Build history of the part. All positions in model axes, mm. A direction names the side the tool comes from. Give positions to 0.01 mm unless a question says otherwise; leave off trailing zeros. Write each loop counter-clockwise with the first axis right and the second up, starting at its lowest first coordinate (ties: lowest second). Pieces come first, ordered by that corner, then holes.
from build123d import *

# Parameters (mm, degrees)
SKETCH1_R           = 14.605
BOSS_EXTRUDE1_DEPTH = 1.524
CUT_EXTRUDE1_DEPTH  = 0.8128
SKETCH4_R           = 0.4445
BOSS_EXTRUDE2_DEPTH = 0.8128
CUT_EXTRUDE2_DEPTH  = 21.670575557
FILLET1_R           = 0.254
FILLET3_R           = 0.254
SNAP_START          = 13.7414
SNAP_HOOK1_DEPTH    = 0.6096
SNAP_START_2        = -0.714869456
SNAP_HOOK1_2_DEPTH  = 1.429738912
SNAP_START_3        = -0.847985215
SNAP_HOOK1_3_DEPTH  = 1.69597043
SNAP_START_4        = 12
SNAP_HOOK1_4_DEPTH  = 4
CIRPATTERN1_COUNT   = 4
SKETCH6_W           = 14.224
SKETCH6_H           = 9.208016637
CUT_EXTRUDE3_DEPTH  = 2.54


with BuildPart() as part:
    # Sketch1 → Boss-Extrude1 (new body)
    with BuildSketch(Plane(origin=(0, 0, 0), x_dir=(1, 0, 0), z_dir=(0, 1, 0))):
        with Locations(Location((0, 0, 0), (0, 0, 270))):
            Circle(SKETCH1_R)
    extrude(amount=BOSS_EXTRUDE1_DEPTH)

    # Sketch3 → Cut-Extrude1 (cut)
    with BuildSketch(Plane(origin=(0, 1.524, 0), x_dir=(1, 0, 0), z_dir=(0, 1, 0))):
        with BuildLine():
            Line((-5.588, -11.967686493), (5.588, -11.967686493))
            ThreePointArc((5.588, -11.967686493), (0, 13.208), (-5.588, -11.967686493))
        make_face()
    extrude(amount=-CUT_EXTRUDE1_DEPTH, mode=Mode.SUBTRACT)

    # Sketch4 → Boss-Extrude2 (add)
    with BuildSketch(Plane(origin=(0, 0.7112, 0), x_dir=(1, 0, 0), z_dir=(0, 1, 0))):
        with Locations(Location((-3.7592, -8.6233, 0), (0, 0, 90))):
            Circle(SKETCH4_R)
        with Locations(Location((3.7592, -8.6233, 0), (0, 0, 90))):
            Circle(SKETCH4_R)
    extrude(amount=BOSS_EXTRUDE2_DEPTH)

    # Sketch5 → Cut-Extrude2 (cut, through all)
    with BuildSketch(Plane(origin=(0, 0.7112, 0), x_dir=(1, 0, 0), z_dir=(0, 1, 0))):
        with BuildLine():
            Line((-9.940854815, -6.887686493), (9.870656967, -6.887686493))
            ThreePointArc((9.870656967, -6.887686493), (-0.035098924, 12.065), (-9.940854815, -6.887686493))
        make_face()
    extrude(amount=-CUT_EXTRUDE2_DEPTH, mode=Mode.SUBTRACT)

    # Fillet1
    fillet1_edges = [part.edges().sort_by_distance(p)[0] for p in [
        (-0.035098924, 0, -12.065),
        (-0.035098924, 0, 6.887686493),
    ]]
    fillet(fillet1_edges, radius=FILLET1_R)

    # Fillet3
    fillet3_edges = [part.edges().sort_by_distance(p)[0] for p in [
        (-3.7592, 1.524, 9.0678),
        (3.7592, 1.524, 9.0678),
    ]]
    fillet(fillet3_edges, radius=FILLET3_R)

    # Snap Hook1: read off the stored shape, not the designer's step
    # Snap Hook1 outline → Snap Hook1 (add)
    with BuildSketch(Plane.XY.offset(SNAP_START)):
        Polygon((-0.847985215, 1.524), (0.847985215, 1.524), (0.635, 5.588), (-0.635, 5.588), align=None)
    snap_hook1 = extrude(amount=SNAP_HOOK1_DEPTH)

    # Snap Hook1 2 outline → Snap Hook1 2 (add)
    with BuildSketch(Plane.YZ.offset(SNAP_START_2)):
        Polygon((1.524, 13.7414), (1.524, 13.335), (5.588, 13.7414), align=None)
        Polygon((4.064, 15.113), (4.064, 14.351), (5.588, 14.351), align=None)
    snap_hook1_2 = extrude(amount=SNAP_HOOK1_2_DEPTH)

    # Snap Hook1 3 outline → Snap Hook1 3 (add)
    with BuildSketch(Plane.YZ.offset(SNAP_START_3)):
        Polygon((1.524, 13.7414), (1.524, 13.335), (5.588, 13.7414), align=None)
    snap_hook1_3 = extrude(amount=SNAP_HOOK1_3_DEPTH)

    # Snap Hook1 4 outline → Snap Hook1 4 (cut)
    with BuildSketch(Plane.XY.offset(SNAP_START_4)):
        Polygon((0.847985215, 1.524), (0.847985215, 7), (0.561000216, 7), (0.635, 5.588), align=None)
        Polygon((-0.635, 5.588), (-0.561000216, 7), (-0.847985215, 7), (-0.847985215, 1.524), align=None)
    snap_hook1_4 = extrude(amount=SNAP_HOOK1_4_DEPTH, mode=Mode.SUBTRACT)

    # CirPattern1: Snap Hook1, Snap Hook1 2, Snap Hook1 3, Snap Hook1 4 ×4 about axis
    cirpattern1_axis = Axis((0, 1.524, 0), (0, 1, 0))
    add([snap_hook1.rotate(cirpattern1_axis, i * 360 / CIRPATTERN1_COUNT) for i in range(1, CIRPATTERN1_COUNT)])
    add([snap_hook1_2.rotate(cirpattern1_axis, i * 360 / CIRPATTERN1_COUNT) for i in range(1, CIRPATTERN1_COUNT)])
    add([snap_hook1_3.rotate(cirpattern1_axis, i * 360 / CIRPATTERN1_COUNT) for i in range(1, CIRPATTERN1_COUNT)])
    add([snap_hook1_4.rotate(cirpattern1_axis, i * 360 / CIRPATTERN1_COUNT) for i in range(1, CIRPATTERN1_COUNT)], mode=Mode.SUBTRACT)

    # Sketch6 → Cut-Extrude3 (cut)
    with BuildSketch(Plane(origin=(0, 0.7112, 0), x_dir=(1, 0, 0), z_dir=(0, 1, 0))):
        with Locations((0, 6.525714051)):
            Rectangle(SKETCH6_W, SKETCH6_H)
    extrude(amount=-CUT_EXTRUDE3_DEPTH, mode=Mode.SUBTRACT)


solid = part.part
(1) Mould opens along Y. For faces 5 (the face through (-3.779, 0.987, 9.067)), 6 (the face through (-14.351, 3, 0)), 7 (the face through (-0.01, 4.837, 14.727)) say: +Y half, -Y half, draft (parallel to the pull), parting line (faces both ways), or undercut.
(2) 3-axis set-ups, long thin cutter, end or side, ignore diameter. For faces 1 (the face through (14.351, 3, 0)), 2 (the face through (13.535, 3.528, 0.012)), 3 (the face through (-0.1, 0.711, -12.4)), 4 (the face through (0, 3, -14.351)): which of +Z, -Z, +X, -X, +Y, -Y reach the whole face in a straight line?
(3) Probe line 1 (X direction, y = 1.1, z = 0) (3 decimals); line 2 (Y direction, x = 0, z = 14.5); line 3 (Y direction, x = 12, z = 8). List the from-to ranges inside material, lowest first.
(4) Saw through at A-A, the plane y = 3.5. List the corners of the cut face in (x, z).
(5) Drop flat-ended pins along their axis: pin 1 (1.9 mm diameter, centred on y = 3, z = 0.5, fed in from +X); pin 2 (14.5 mm diameter, centred on x = -4, z = -6, fed in from +Y); pin 3 (0.6 mm diameter, centred on y = 0.5, z = -10.5, fed in from -X). Give the stop position or say it passes through.
Computed values:
1. face 5: draft
1. face 6: undercut
1. face 7: +Y half
2. face 1: +Z, -Z, +X
2. face 2: +Z, -Z, +Y
2. face 3: +Y
2. face 4: -Z, +X, -X
3. line 1: x = -14.605 to -13.208, 13.208 to 14.605
3. line 2: y = 0 to 1.52, 4.06 to 5.29
3. line 3: y = 0 to 1.52
4. outline: (-14.35, -0.74) - (-13.53, -0.74) - (-13.53, 0.74) - (-14.35, 0.74) - close; (-0.74, -14.35) - (0.74, -14.35) - (0.74, -13.53) - (-0.74, -13.53) - close; (-0.74, 13.53) - (0.74, 13.53) - (0.74, 14.35) - (-0.74, 14.35) - close; (13.53, -0.74) - (14.35, -0.74) - (14.35, 0.74) - (13.53, 0.74) - close
5. pin 1: stops at x = 14.35
5. pin 2: stops at y = 1.52
5. pin 3: stops at x = -10.45
